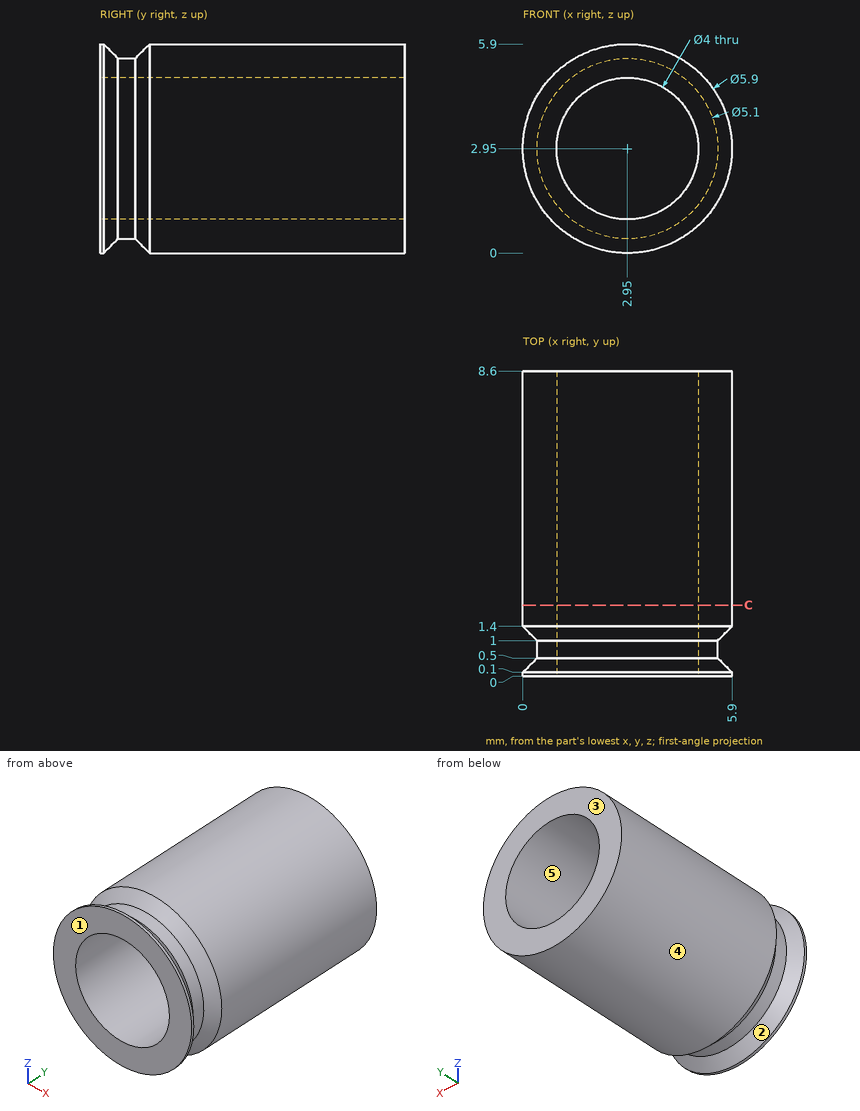
Verification items for this drawing (mm, ordinates from the low corner). A direction names the side the tool comes from. Coordinates: 2 decimals unless noted, no trailing zeros. Write each loop counter-clockwise with the first axis right and the second up, starting at its lowest first coordinate (ties: lowest second). Pieces come first, ordered by that corner, then holes. Notation, with made-up numbers: M -21.75,16 L 22.25,16 A12 ccw 22.25,37 Z; hole C 17.25,1 d5. An arc over 180 degrees is marked long. Answer as a JSON object with one key per item and string values. Group by question number.
(1) Cross-section at C-C, the plane y = 2. Record the cut outline in (x, z), and give its area (3 significant figures).
(2) Gauge pin test, flat ends, axial feed: pin 1 (2.5 mm diameter, centred on x = 2.95, z = 2.95, fed in from -Y); pin 2 (3 mm diameter, centred on x = 2, y = 4.5, fed in from -Z). Record the tip position at first contact, or that the pin passes through.
(3) Tool access check on the marked faces 1 and 2. Record the directions out of +Z, -Z, +X, -X, +Y, -Y that give a thin tool (end or side, any length) a straight path to the whole face; none if there is none.
(4) Material ranges on line 1 (X direction, y = 6, z = 3.05); line 2 (Y direction, x = 0.75, z = 4.5); line 3 (X direction, y = 3, z = 4.45), recorded low to high.
(5) Release check for a two-part mould opening along X. For the marked faces 3, 4 and 5 record: +X half, -X half, draft (parallel to the pull), parting line (faces both ways), or undercut.
Reply:
{
 "1": {"outline": "C 2.95,2.95 d5.9; hole C 2.95,2.95 d4", "area": "14.8 mm²"},
 "2": {"pin 1": "through", "pin 2": "z = 0"},
 "3": {"face 1": "+Z, -Z, +X, -X, -Y", "face 2": "none"},
 "4": {"line 1": "0 to 0.95, 4.95 to 5.9", "line 2": "0 to 0.36, 1.14 to 8.6", "line 3": "0.41 to 1.63, 4.27 to 5.49"},
 "5": {"face 3": "draft", "face 4": "parting line", "face 5": "undercut"}
}
